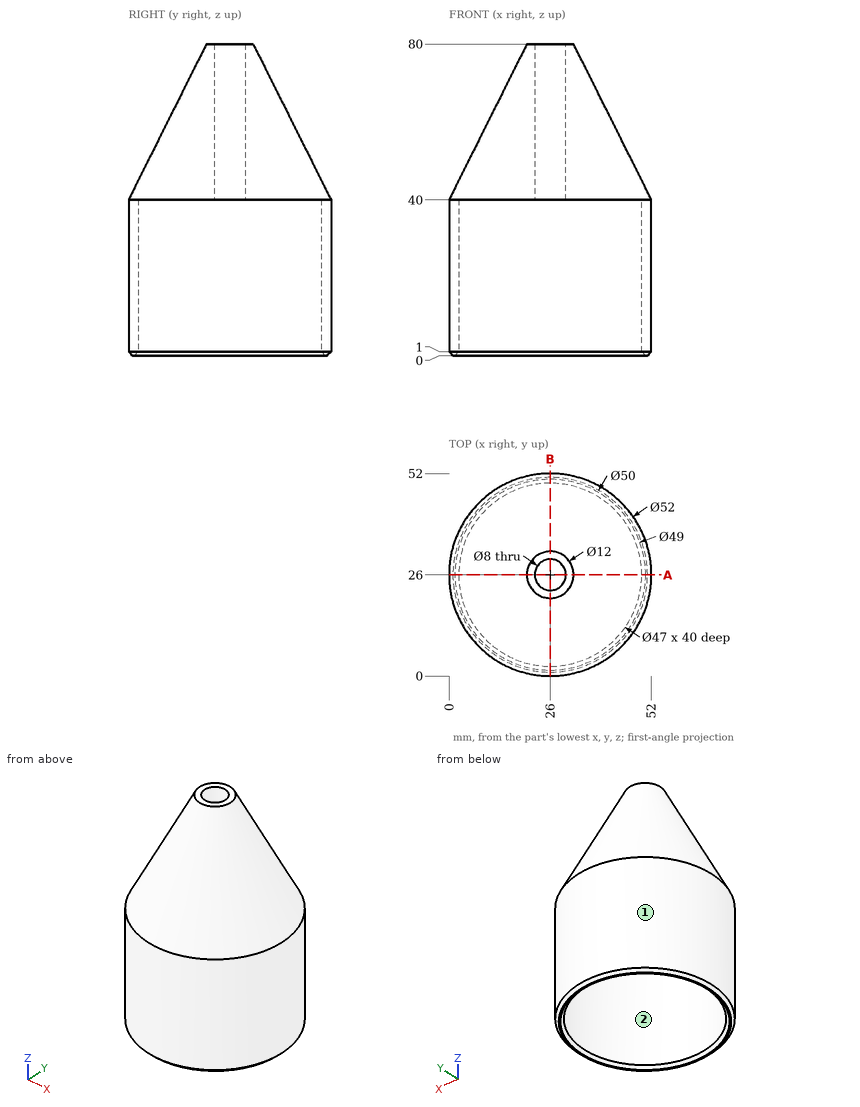
Design review of the part shown in the three views and the two pictorial views. Dimensions are in mm from the part's minimum x, y and z. Give positions to 0.01 mm unless a question says otherwise; leave off trailing zeros. Write each loop counter-clockwise with the first axis right and the second up, starting at its lowest first coordinate (ties: lowest second). Pieces come first, ordered by that corner, then holes. Notation, with made-up numbers: M 16,4 L 37,4 A21 cw 37,24 Z; hole C 54,58 d6. An arc over 180 degrees is marked long. One line per item, written item: value.
1) Take a section at A-A, the plane y = 26. Write out the cut boundary in (x, z), then the cut area to 3 significant figures.
Results are:
outline: M 0,1 L 1,0 L 1.5,0 L 2.5,1 L 2.5,40 L 22,40 L 22,80 L 20,80 L 0,40 Z; M 30,40 L 49.5,40 L 49.5,1 L 50.5,0 L 51,0 L 52,1 L 52,40 L 32,80 L 30,80 Z
area: 1,160 mm²
2) For line 1 (Y direction, x = 26, z = 11); line 2 (Y direction, x = 47, z = 39); line 3 (X direction, y = 37, z = 36.5), list the stretches that pass through material, from the lowest coordinate up. Write a range as from..to.
Results are:
line 1: y = 0..2.5, 49.5..52
line 2: y = 10.67..15.45, 36.55..41.33
line 3: x = 2.44..5.23, 46.77..49.56
3) For P1, Ø5, axis at x = 29, z = 67, coming from the -Y side; P2, Ø12, axis at x = 22.5, z = 12.5, coming from the +Y side; P3, Ø3, axis at y = 18, z = 29.5, coming from the -X side, all flat-tipped, find the tip position at first contact; note any pin that passes through.
Results are:
P1: stops at y = 12.49
P2: stops at y = 52
P3: stops at x = 0.83
4) The part is to be moulded in two halves that separate along X. For the marked faces 1 and 2, say which applies: +X half, -X half, draft (parallel to the pull), parting line (faces both ways), or undercut.
Results are:
face 1: parting line
face 2: undercut
